from build123d import *

# Parameters (mm, degrees)
ESQUISSE2_R              = 58
BOSS_EXTRU_2_DEPTH       = 30
ENL_V_MAT_EXTRU_2_DEPTH  = 28
ENL_V_MAT_EXTRU_3_DEPTH  = 28
ENL_V_MAT_EXTRU_8_DEPTH  = 28
ENL_V_MAT_EXTRU_10_DEPTH = 28
ESQUISSE18_R             = 3
ENL_V_MAT_EXTRU_11_DEPTH = 30
ESQUISSE21_R             = 3.5
ENL_V_MAT_EXTRU_13_DEPTH = 28
ENL_V_START              = -10
ESQUISSE22_R             = 3.5
ENL_V_MAT_EXTRU_14_DEPTH = 10


with BuildPart() as part:
    # Esquisse2 → Boss.-Extru.2 (new body)
    with BuildSketch(Plane(origin=(0, 0, 0), x_dir=(1, 0, 0), z_dir=(0, 1, 0))):
        with Locations(Location((0, 0, 0), (0, 0, 270))):
            Circle(ESQUISSE2_R)
    extrude(amount=BOSS_EXTRU_2_DEPTH)

    # Esquisse3 → Enlèv. mat.-Extru.2 (cut)
    with BuildSketch(Plane(origin=(0, 30, 0), x_dir=(1, 0, 0), z_dir=(0, 1, 0))):
        with BuildLine():
            Line((-55.99137867, 1), (-1, 1))
            Line((-1, 1), (-1, 55.940862442))
            ThreePointArc((-1, 55.940862442), (-39.531080805, 39.515969353), (-55.99137867, 1))
        make_face()
    extrude(amount=-ENL_V_MAT_EXTRU_2_DEPTH, mode=Mode.SUBTRACT)

    # Esquisse5 → Enlèv. mat.-Extru.3 (cut)
    with BuildSketch(Plane(origin=(0, 30, 0), x_dir=(1, 0, 0), z_dir=(0, 1, 0))):
        with BuildLine():
            Line((0.999998069, 55.991388398), (0.999998069, 1.000009729))
            Line((0.999998069, 1.000009729), (55.940860512, 1.000009729))
            ThreePointArc((55.940860512, 1.000009729), (39.515967422, 39.531090534), (0.999998069, 55.991388398))
        make_face()
    extrude(amount=-ENL_V_MAT_EXTRU_3_DEPTH, mode=Mode.SUBTRACT)

    # Esquisse14 → Enlèv. mat.-Extru.8 (cut)
    with BuildSketch(Plane(origin=(0, 30, 0), x_dir=(1, 0, 0), z_dir=(0, 1, 0))):
        with BuildLine():
            Line((-1.000000805, -55.991378782), (-1.000000805, -1.000000112))
            Line((-1.000000805, -1.000000112), (-55.940863247, -1.000000112))
            ThreePointArc((-55.940863247, -1.000000112), (-39.515970158, -39.531080917), (-1.000000805, -55.991378782))
        make_face()
    extrude(amount=-ENL_V_MAT_EXTRU_8_DEPTH, mode=Mode.SUBTRACT)

    # Esquisse17 → Enlèv. mat.-Extru.10 (cut)
    with BuildSketch(Plane(origin=(0, 30, 0), x_dir=(1, 0, 0), z_dir=(0, 1, 0))):
        with BuildLine():
            Line((55.991361526, -0.999992166), (0.999998069, -1.000000112))
            Line((0.999998069, -1.000000112), (0.999982856, -55.940854608))
            ThreePointArc((0.999982856, -55.940854608), (39.531063661, -39.515961519), (55.991361526, -0.999992166))
        make_face()
    extrude(amount=-ENL_V_MAT_EXTRU_10_DEPTH, mode=Mode.SUBTRACT)

    # Esquisse18 → Enlèv. mat.-Extru.11 (cut)
    with BuildSketch(Plane.XZ):
        with Locations(Location((0, 0, 0), (0, 0, 270))):
            Circle(ESQUISSE18_R)
    extrude(amount=-ENL_V_MAT_EXTRU_11_DEPTH, mode=Mode.SUBTRACT)

    # Esquisse21 → Enlèv. mat.-Extru.13 (cut)
    with BuildSketch(Plane(origin=(0, 2, 0), x_dir=(1, 0, 0), z_dir=(0, 1, 0))):
        Circle(ESQUISSE21_R)
    extrude(amount=ENL_V_MAT_EXTRU_13_DEPTH, mode=Mode.SUBTRACT)

    # Esquisse22 → Enlèv. mat.-Extru.14 (cut)
    with BuildSketch(Plane(origin=(0, 2, 0), x_dir=(1, 0, 0), z_dir=(0, 1, 0)).offset(ENL_V_START)):
        with Locations(Location((0, 0, 0), (0, 0, 73.398483382))):
            Circle(ESQUISSE22_R)
    extrude(amount=ENL_V_MAT_EXTRU_14_DEPTH, mode=Mode.SUBTRACT)


solid = part.part
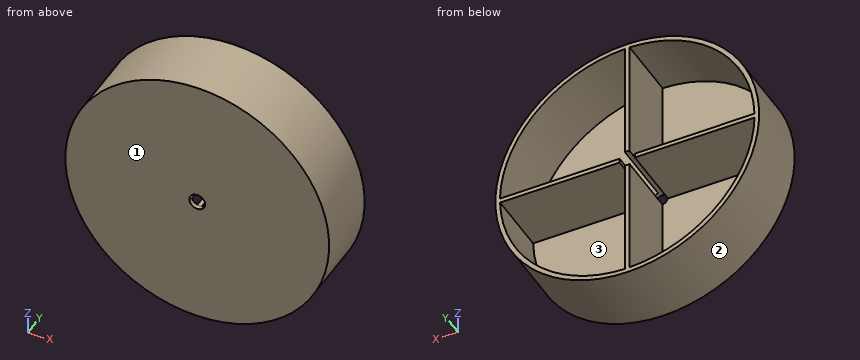
Input: part model. Units: mm. Frame: model coordinates. Face numbers are marked on the shaded views. Round coordinates to 2 decimals unless told otherwise and drop trailing zeros. Loops run counter-clockwise (first coordinate to the right, second up) from the corner with the lowest first, then second, coordinate; pieces in that order, holes last. Notation, with made-up numbers: (6.5, 82) -> (50.5, 82) arc R18 ccw to (50.5, 115) -> close; hole circle Ø6 at (-31.5, 57). An arc over 180 degrees is marked (long way). Answer as a JSON object with one key per item and string values. Group by question number.
1) Section query B-B on x = 48. Output: boundary loops of the cut face in (y, z), plus the area to 3 significant figures.
2) Pin query (flat end, axial travel): pin 1 (12 mm diameter, centred on y = 15.5, z = -31.5, fed in from +X); pin 2 (8 mm diameter, centred on x = 29.5, z = -34, fed in from +Y); pin 3 (14 mm diameter, centred on x = 39.5, y = 10, fed in from -Z). Return the tip coordinate at first contact, or that it passes through.
3) Draft query along Z for the marked faces 1, 2 and 3. Return one class per face: +Z half, -Z half, draft (parallel to the pull), parting line (faces both ways), or undercut.
4) Section query A-A on y = 11.25. Output: boundary loops of the cut face in (x, z).
5) Section query C-C on z = -32.5. Output: boundary loops of the cut face in (x, y).
6) Ray query, L1, parallel to X at y = 15.75, z = 0; L2, parallel to Z at x = -43, y = 3.25; L3, parallel to X at y = 26.5, z = 37. Return the intervals inside material, ascending.
Reply:
{
 "1": {"outline": "(0, -32.56) -> (30, -32.56) -> (30, -28.64) -> (2, -28.64) -> (2, -1) -> (30, -1) -> (30, 1) -> (2, 1) -> (2, 28.67) -> (30, 28.67) -> (30, 32.56) -> (0, 32.56) -> close", "area": "405 mm2"},
 "2": {"pin 1": "stops at x = 52.09", "pin 2": "stops at y = 2", "pin 3": "stops at z = -48.04"},
 "3": {"face 1": "draft", "face 2": "parting line", "face 3": "undercut"},
 "4": {"outline": "circle Ø116 at (0, 0); hole (-55.99, -1) arc R56.18 ccw to (-1, -55.94) -> (-1, -3.35) arc R3.5 ccw to (1, -3.35) -> (1, -55.99) arc R56.18 ccw to (55.94, -1) -> (3.35, -1) arc R3.5 ccw to (3.35, 1) -> (55.99, 1) arc R56.18 ccw to (1, 55.94) -> (1, 3.35) arc R3.5 ccw to (-1, 3.35) -> (-1, 55.99) arc R56.18 ccw to (-55.94, 1) -> (-3.35, 1) arc R3.5 ccw to (-3.35, -1) -> close"},
 "5": {"outline": "(-48.04, 0) -> (48.04, 0) -> (48.04, 30) -> (45.47, 30) -> (45.47, 2) -> (1, 2) -> (1, 30) -> (-1, 30) -> (-1, 2) -> (-45.49, 2) -> (-45.49, 30) -> (-48.04, 30) -> close"},
 "6": {"L1": "x = -58 to -3.5, 3.5 to 58", "L2": "z = -38.92 to -35.72, -1 to 1, 35.71 to 38.92", "L3": "x = -44.67 to -41.89, -1 to 1, 41.9 to 44.67"}
}
